The model under review builds one solid part; all positions refer to its coordinate system, in mm. Coordinates: 2 decimals unless noted, no trailing zeros. Write each loop counter-clockwise with the first axis right and the second up, starting at its lowest first coordinate (ties: lowest second). Pieces come first, ordered by that corner, then holes. Notation, with made-up numbers: (68, 2) - (116, 2) arc R30 ccw to (116, 33) - close; hole circle Ø7 at (6, 12.5). An arc over 180 degrees is marked (long way). Put each result on its own line as item: value. Start each with the question number.
Item 1: For pin 1 (1.6 mm diameter, centred on x = 5.5, z = 2.5, fed in from -Y), flat-tipped, find the tip position at first contact; note if it passes through.
Item 2: Consider section B-B on z = 1.5. Give the boundary of the cut face in (x, y), then the cut area to 3 significant figures.
Item 3: Mouldability with a two-part tool opening along Z and no side actions: class faces 1 (the face through (-2.41, -11.24, 4.3)), 2 (the face through (9.47, -7, 2)), 3 (the face through (-2.33, -11.24, 0.62)), 4 (the face through (0.48, -8.22, 3.36)) as pulls with the +Z half, pulls with the -Z half, needs draft (parallel to the pull), parting line crosses it, or undercut.
Item 4: Consider section C-C on y = -9.5. Give the boundary of the cut face in (x, z), then the cut area to 3 significant figures.
Item 5: Consider section D-D on z = 3.2. Give the boundary of the cut face in (x, y).
Item 6: To check wall thickness, follow L1, parallel to X at y = -10.75, z = 2.65; L2, parallel to X at y = -7.25, z = 2.25; L3, parallel to Z at x = 6.25, y = -8.5. State the ranges of each line that lie inside material, in increasing order. Write a range as [from, to].
Item 7: Consider section A-A on x = 3.5. Give the boundary of the cut face in (y, z), then the cut area to 3 significant figures.
```python
from build123d import *

# Parameters (mm, degrees)
F1_DEPTH = 5
F3_SIZE  = 1
F4_R     = 0.7470588235
F5_DEPTH = 7.5


# Not quite as in the source:
# - a feature names something its author has since deleted; it is built from what else it names


with BuildPart() as f1:
    # F0 (on Top) → F1 (new body)
    with BuildSketch(Plane.XY):
        Polygon((9.4699421152, -1.9223576039), (-3.0300578848, -1.9223576039), (-3.0300578848, -6.9223576039), (-3.0300578848, -11.9223576039), (9.4699421152, -11.9223576039), align=None)
    extrude(amount=F1_DEPTH)

    # F3
    f3_edges = [f1.edges().sort_by_distance(p)[0] for p in [
        (3.219942, -11.922358, 5),
        (9.469942, -6.922358, 5),
        (-3.030058, -1.922358, 2.5),
        (-3.030058, -11.922358, 2.5),
        (9.469942, -11.922358, 2.5),
        (9.469942, -6.922358, 0),
        (3.219942, -11.922358, 0),
        (9.469942, -1.922358, 2.5),
        (-3.030058, -6.922358, 5),
        (3.219942, -1.922358, 5),
        (3.219942, -1.922358, 0),
        (-3.030058, -6.922358, 0),
    ]]
    chamfer(f3_edges, length=F3_SIZE)

    # F4 (on face) → F5 (cut)
    with BuildSketch(Plane.XZ.offset(11.9223576039)):
        with Locations((0.5804465618, 2.6189445052)):
            Circle(F4_R)
        with Locations((5.8481891174, 2.6189445052)):
            Circle(F4_R)
    extrude(amount=-F5_DEPTH, mode=Mode.SUBTRACT)


solid = f1.part
```
Report:
1. pin 1: y = -11.92
2. outline: (-3.03, -10.92) - (-2.03, -11.92) - (8.47, -11.92) - (9.47, -10.92) - (9.47, -2.92) - (8.47, -1.92) - (-2.03, -1.92) - (-3.03, -2.92) - close
2. area: 123 mm²
3. face 1: pulls with the +Z half
3. face 2: needs draft
3. face 3: pulls with the -Z half
3. face 4: undercut
4. outline: (-3.03, 1) - (-2.03, 0) - (8.47, 0) - (9.47, 1) - (9.47, 4) - (8.47, 5) - (-2.03, 5) - (-3.03, 4) - close; hole circle Ø1.49 at (0.58, 2.62); hole circle Ø1.49 at (5.85, 2.62)
4. area: 57.0 mm²
5. outline: (-3.03, -10.92) - (-2.03, -11.92) - (0.11, -11.92) - (0.11, -4.42) - (1.05, -4.42) - (1.05, -11.92) - (5.38, -11.92) - (5.38, -4.42) - (6.32, -4.42) - (6.32, -11.92) - (8.47, -11.92) - (9.47, -10.92) - (9.47, -2.92) - (8.47, -1.92) - (-2.03, -1.92) - (-3.03, -2.92) - close
6. L1: [-3.03, -0.17], [1.33, 5.1], [6.59, 9.47]
6. L2: [-3.03, -0.07], [1.23, 5.2], [6.5, 9.47]
6. L3: [0, 1.99], [3.25, 5]
7. outline: (-11.92, 1) - (-10.92, 0) - (-2.92, 0) - (-1.92, 1) - (-1.92, 4) - (-2.92, 5) - (-10.92, 5) - (-11.92, 4) - close
7. area: 48.0 mm²
